Verification items for the finished model (mm, model axes). Coordinates: 2 decimals unless noted, no trailing zeros. Order: outer loops, then holes, each group sorted by start corner. A loop starts at its lowest first (then second) coordinate and runs counter-clockwise, first axis right, second up. Notation, with made-up numbers: M 28.5,85 L 65.5,85 A8 cw 65.5,97 Z; hole C -22.5,72 d3. An arc over 180 degrees is marked long. Return JSON: item names as keys, results as strings.
```python
from build123d import *

# Parameters (mm, degrees)
F0_W     = 6.35
F0_H     = 25.4
F1_DEPTH = 1.5875
F2_R     = 2.21245533
F3_DEPTH = 0.3560978221


with BuildPart() as f1:
    # F0 (on Front) → F1 (new body)
    with BuildSketch(Plane.XZ):
        Rectangle(F0_W, F0_H)
    extrude(amount=F1_DEPTH)

    # F2 (on face) → F3 (join)
    with BuildSketch(Plane.XZ.offset(1.5875)):
        with Locations((0, -9.151885286)):
            Circle(F2_R)
        with BuildLine():
            ThreePointArc((-0.5292957498, 12.7), (-1.3777807408, 8.7779312566), (2.2310145846, 10.5326808989))
            ThreePointArc((2.2310145846, 10.5326808989), (1.7547496423, 11.9104616397), (0.5292957498, 12.7))
            Line((0.5292957498, 12.7), (-0.5292957498, 12.7))
        make_face()
    extrude(amount=F3_DEPTH)


solid = f1.part
```
Q1. Cross-section at A-A, the plane x = 0. Record the boundary of the cut face in (y, z).
Values:
{"outline": "M -1.94,-11.36 L -1.59,-11.36 L -1.59,-12.7 L 0,-12.7 L 0,12.7 L -1.94,12.7 L -1.94,8.3 L -1.59,8.3 L -1.59,-6.94 L -1.94,-6.94 Z"}
Q2. Draft check along Z on faces 1 (the face through (-0.29, -1.76, -6.96)), 2 (the face through (0, -1, 12.7)), 3 (the face through (0, 0, 0)), 4 (the face through (0, -1.588, 0)). Enter one of: pulls with the +Z half, pulls with the -Z half, needs draft (parallel to the pull), parting line crosses it, or undercut.
Values:
{"face 1": "undercut", "face 2": "pulls with the +Z half", "face 3": "needs draft", "face 4": "undercut"}
Q3. Cross-section at B-B, the plane z = -4.75. Record the boundary of the cut face in (x, y) (1 decimal), and give its area (3 significant figures).
Values:
{"outline": "M -3.2,-1.6 L 3.2,-1.6 L 3.2,0 L -3.2,0 Z", "area": "10.1 mm^2"}
Q4. Cross-section at C-C, the plane x = 2. Record the boundary of the cut face in (y, z), and give its area (3 significant figures).
Values:
{"outline": "M -1.94,-10.1 L -1.59,-10.1 L -1.59,-12.7 L 0,-12.7 L 0,12.7 L -1.59,12.7 L -1.59,11.52 L -1.94,11.52 L -1.94,9.54 L -1.59,9.54 L -1.59,-8.21 L -1.94,-8.21 Z", "area": "41.7 mm^2"}
Q5. Material ranges on line 1 along Y through (x, z) = (1.5, -0.5); line 2 along Z through (x, y) = (0.5, -1.8); line 3 along X through (y, z) = (-1.65, -8), recorded low to high.
Values:
{"line 1": "-1.59 to 0", "line 2": "-11.31 to -7, 8.36 to 12.7", "line 3": "-1.89 to 1.89"}
Q6. Go/stop test with a flat-tipped pin: pin 1 (3 mm diameter, centred on x = -0.5, z = 5.5, fed in from -Y). Record where the tip stops, or that it passes through.
Values:
{"pin 1": "y = -1.59"}
